Verification items for the finished model (mm, model axes). A direction names the side the tool comes from. Coordinates: 2 decimals unless noted, no trailing zeros. Loops run counter-clockwise (first coordinate to the right, second up) from the corner with the lowest first, then second, coordinate; pieces in that order, holes last. Notation, with made-up numbers: (28, 13.5) -> (43, 13.5) arc R27 cw to (43, 41.5) -> close; hole circle Ø6 at (-36, 62). An arc over 180 degrees is marked (long way). Answer as a JSON object with one key per item and string values. Group by question number.
Q1. Cross-section at D-D on z = 85.5. Record the boundary of the cut face in (x, y), and give its area (3 significant figures).
Q2. Cross-section at C-C on x = 63. Record the boundary of the cut face in (y, z).
Q3. Scan lines: L1, parallel to Y at x = 109.5, z = 40; L2, parallel to Z at x = 83, y = 8.4; L3, parallel to Z at x = 20, y = 6. Record each from-to range of solid material in increasing order.
Q4. Set-up check for faces 1 (the flat face through (72.5, 7, 76)), 2 (the flat face through (5, 47, 95)), 3 (the cylindrical face through (108, 46, 40)), 4 (the flat face through (106, 53, 8)): record each of +Z, -Z, +X, -X, +Y, -Y from which the full face is reachable in a straight line by a thin tool's end or side.
Q5. Cross-section at B-B on x = 83. Record the boundary of the cut face in (y, z).
Q6. Gauge pin test, flat ends, axial feed: pin 1 Ø1.2 at (x, y) = (4, 54) entering from -Z; pin 2 Ø1.2 at (x, y) = (107.5, 54.5) entering from +Z; pin 3 Ø8 at (x, z) = (50.5, 27.5) entering from +Y. Record the tip position at first contact, or that the pin passes through.
Q7. Cross-section at A-A on y = 38. Record the boundary of the cut face in (x, z), and give its area (3 significant figures).
Q8. Release check for a two-part mould opening along Y. For faces 5 (the cylindrical face through (108, 32, 40)), 6 (the flat face through (80, 6, 25)), 7 (the flat face through (68, 5, 13.5)), 8 (the flat face through (5, 80, 49)) record: released by +Y, released by -Y, zero draft, split by the parting line, or undercut.
```python
from build123d import *

# Parameters (mm, degrees)
BOX003_W                = 37
BOX003_H                = 7
BOX003_DEPTH            = 7
CYLINDER001_R           = 2
CYLINDER001_DEPTH       = 20
CYLINDER001_ROLL_ANGLE  = 90
ARRAY001_X_COUNT        = 2
ARRAY001_X_PITCH        = 28
ARRAY001_Z_COUNT        = 2
ARRAY001_Z_PITCH        = 50
BOX004_W                = 13
BOX004_H                = 12
BOX004_DEPTH            = 3.5
ARRAY003_X_COUNT        = 2
ARRAY003_X_PITCH        = 102
ARRAY003_Z_COUNT        = 2
ARRAY003_Z_PITCH        = 90.5
BOX002_W                = 37
BOX002_H                = 7
BOX002_DEPTH            = 7
BOX005_W                = 4
BOX005_H                = 6
BOX005_DEPTH            = 11
CYLINDER004_R           = 2
CYLINDER004_DEPTH       = 11
CYLINDER003_R           = 2
CYLINDER003_DEPTH       = 11
ARRAY004_X_COUNT        = 2
ARRAY004_X_PITCH        = 103
ARRAY004_Z_COUNT        = 2
ARRAY004_Z_PITCH        = 91
CYLINDER007_R           = 12
CYLINDER007_DEPTH       = 12
CYLINDER007_PITCH_ANGLE = 90
CYLINDER006_R           = 2.25
CYLINDER006_DEPTH       = 12
CYLINDER006_PITCH_ANGLE = 90
ARRAY006_Y_COUNT        = 2
ARRAY006_Y_PITCH        = 31
ARRAY006_Z_COUNT        = 2
ARRAY006_Z_PITCH        = 31
CYLINDER005_R           = 12
CYLINDER005_DEPTH       = 12
CYLINDER005_PITCH_ANGLE = 90
ARRAY005_Y_COUNT        = 2
ARRAY005_Y_PITCH        = 31
ARRAY005_Z_COUNT        = 2
ARRAY005_Z_PITCH        = 31
CYLINDER002_R           = 2
CYLINDER002_DEPTH       = 20
CYLINDER002_PITCH_ANGLE = 90
ARRAY002_Y_COUNT        = 4
ARRAY002_Y_PITCH        = 14
ARRAY002_Z_COUNT        = 4
ARRAY002_Z_PITCH        = 20
CYLINDER_R              = 2.5
CYLINDER_DEPTH          = 20
CYLINDER_ROLL_ANGLE     = 90
ARRAY_X_COUNT           = 2
ARRAY_X_PITCH           = 73
ARRAY_Z_COUNT           = 2
ARRAY_Z_PITCH           = 80
BOX001_W                = 8
BOX001_H                = 20
BOX001_DEPTH            = 24
BOX_W                   = 8
BOX_H                   = 20
BOX_DEPTH               = 24
EXTRUDE001_DEPTH        = 100
FILLET_R                = 1.5


with BuildPart() as h_bearing_up_h:
    # Box003 → Box003 (new body)
    with BuildSketch(Plane(origin=(50, -1, 72), x_dir=(1, 0, 0), z_dir=(0, 0, 1))):
        with Locations((18.5, 3.5)):
            Rectangle(BOX003_W, BOX003_H)
    extrude(amount=BOX003_DEPTH)


with BuildPart() as h_bearing_bolt:
    # Cylinder001 → Cylinder001 (new body)
    with BuildSketch(Plane.XY):
        Circle(CYLINDER001_R)
    extrude(amount=CYLINDER001_DEPTH)


with BuildPart() as h_bearing_bolt_1:
    # Cylinder001 roll: moved
    add(h_bearing_bolt.part.rotate(Axis((0, 0, 0), (1, 0, 0)), CYLINDER001_ROLL_ANGLE))


with BuildPart() as h_bearing_bolt_2:
    # Cylinder001 placement: moved
    add(h_bearing_bolt_1.part.moved(Location((55, 15, 25.5))))

    # Array001 X: h_bearing_bolt ×2


with BuildPart() as h_bearing_bolt_3:
    add(h_bearing_bolt_2.part)
    with Locations(*[(i * ARRAY001_X_PITCH, 0, 0) for i in range(1, ARRAY001_X_COUNT)]):
        add(h_bearing_bolt_2.part)

    # Array001 Z: h_bearing_bolt ×2


with BuildPart() as h_bearing_bolt_4:
    add(h_bearing_bolt_3.part)
    with Locations(*[(0, 0, i * ARRAY001_Z_PITCH) for i in range(1, ARRAY001_Z_COUNT)]):
        add(h_bearing_bolt_3.part)


with BuildPart() as h_nut_union001:
    # Box004 → Box004 (new body)
    with BuildSketch(Plane(origin=(-1, 47, 3), x_dir=(1, 0, 0), z_dir=(0, 0, 1))):
        with Locations((6.5, 6)):
            Rectangle(BOX004_W, BOX004_H)
    extrude(amount=BOX004_DEPTH)

    # Array003 X: h_nut_union001 ×2


with BuildPart() as h_nut_union001_1:
    add(h_nut_union001.part)
    with Locations(*[(i * ARRAY003_X_PITCH, 0, 0) for i in range(1, ARRAY003_X_COUNT)]):
        add(h_nut_union001.part)

    # Array003 Z: h_nut_union001 ×2


with BuildPart() as h_nut_union001_2:
    add(h_nut_union001_1.part)
    with Locations(*[(0, 0, i * ARRAY003_Z_PITCH) for i in range(1, ARRAY003_Z_COUNT)]):
        add(h_nut_union001_1.part)


with BuildPart() as h_bearing_dn_h:
    # Box002 → Box002 (new body)
    with BuildSketch(Plane(origin=(50, -1, 22), x_dir=(1, 0, 0), z_dir=(0, 0, 1))):
        with Locations((18.5, 3.5)):
            Rectangle(BOX002_W, BOX002_H)
    extrude(amount=BOX002_DEPTH)


with BuildPart() as h_bolt_union002:
    # Box005 → Box005 (new body)
    with BuildSketch(Plane(origin=(3, 50, -1), x_dir=(1, 0, 0), z_dir=(0, 0, 1))):
        with Locations((2, 3)):
            Rectangle(BOX005_W, BOX005_H)
    extrude(amount=BOX005_DEPTH)


with BuildPart() as h_bolt_union001:
    # Cylinder004 → Cylinder004 (new body)
    with BuildSketch(Plane(origin=(5, 56, -1), x_dir=(1, 0, 0), z_dir=(0, 0, 1))):
        Circle(CYLINDER004_R)
    extrude(amount=CYLINDER004_DEPTH)


with BuildPart() as h_bolt_union004:
    # Cylinder003 → Cylinder003 (new body)
    with BuildSketch(Plane(origin=(5, 50, -1), x_dir=(1, 0, 0), z_dir=(0, 0, 1))):
        Circle(CYLINDER003_R)
    extrude(amount=CYLINDER003_DEPTH)

    # Fusion: union h_bolt_union002, h_bolt_union001
    add(h_bolt_union002.part)
    add(h_bolt_union001.part)

    # Array004 X: h_bolt_union004 ×2


with BuildPart() as h_bolt_union004_1:
    add(h_bolt_union004.part)
    with Locations(*[(i * ARRAY004_X_PITCH, 0, 0) for i in range(1, ARRAY004_X_COUNT)]):
        add(h_bolt_union004.part)

    # Array004 Z: h_bolt_union004 ×2


with BuildPart() as h_bolt_union004_2:
    add(h_bolt_union004_1.part)
    with Locations(*[(0, 0, i * ARRAY004_Z_PITCH) for i in range(1, ARRAY004_Z_COUNT)]):
        add(h_bolt_union004_1.part)


with BuildPart() as h_motor_axis001:
    # Cylinder007 → Cylinder007 (new body)
    with BuildSketch(Plane.XY):
        Circle(CYLINDER007_R)
    extrude(amount=CYLINDER007_DEPTH)


with BuildPart() as h_motor_axis001_1:
    # Cylinder007 pitch: moved
    add(h_motor_axis001.part.rotate(Axis((0, 0, 0), (0, 1, 0)), CYLINDER007_PITCH_ANGLE))


with BuildPart() as h_motor_axis001_2:
    # Cylinder007 placement: moved
    add(h_motor_axis001_1.part.moved(Location((-1, 60, 25))))


with BuildPart() as h_bolt_motor:
    # Cylinder006 → Cylinder006 (new body)
    with BuildSketch(Plane.XY):
        Circle(CYLINDER006_R)
    extrude(amount=CYLINDER006_DEPTH)


with BuildPart() as h_bolt_motor_1:
    # Cylinder006 pitch: moved
    add(h_bolt_motor.part.rotate(Axis((0, 0, 0), (0, 1, 0)), CYLINDER006_PITCH_ANGLE))


with BuildPart() as h_bolt_motor_2:
    # Cylinder006 placement: moved
    add(h_bolt_motor_1.part.moved(Location((-1, 44.5, 9.5))))


with BuildPart() as h_holes_motor_dn:
    # Array006 base: copy of h_bolt_motor
    add(h_bolt_motor_2.part)

    # Array006 Y: h_holes_motor_dn ×2


with BuildPart() as h_holes_motor_dn_1:
    add(h_holes_motor_dn.part)
    with Locations(*[(0, i * ARRAY006_Y_PITCH, 0) for i in range(1, ARRAY006_Y_COUNT)]):
        add(h_holes_motor_dn.part)

    # Array006 Z: h_holes_motor_dn ×2


with BuildPart() as h_holes_motor_dn_2:
    add(h_holes_motor_dn_1.part)
    with Locations(*[(0, 0, i * ARRAY006_Z_PITCH) for i in range(1, ARRAY006_Z_COUNT)]):
        add(h_holes_motor_dn_1.part)

    # Fusion002: union h_motor_axis001
    add(h_motor_axis001_2.part)


with BuildPart() as h_motor_axis:
    # Cylinder005 → Cylinder005 (new body)
    with BuildSketch(Plane.XY):
        Circle(CYLINDER005_R)
    extrude(amount=CYLINDER005_DEPTH)


with BuildPart() as h_motor_axis_1:
    # Cylinder005 pitch: moved
    add(h_motor_axis.part.rotate(Axis((0, 0, 0), (0, 1, 0)), CYLINDER005_PITCH_ANGLE))


with BuildPart() as h_motor_axis_2:
    # Cylinder005 placement: moved
    add(h_motor_axis_1.part.moved(Location((-1, 60, 25))))


with BuildPart() as h_holes_motor_up:
    # Array005 base: copy of h_bolt_motor
    add(h_bolt_motor_2.part)

    # Array005 Y: h_holes_motor_up ×2


with BuildPart() as h_holes_motor_up_1:
    add(h_holes_motor_up.part)
    with Locations(*[(0, i * ARRAY005_Y_PITCH, 0) for i in range(1, ARRAY005_Y_COUNT)]):
        add(h_holes_motor_up.part)

    # Array005 Z: h_holes_motor_up ×2


with BuildPart() as h_holes_motor_up_2:
    add(h_holes_motor_up_1.part)
    with Locations(*[(0, 0, i * ARRAY005_Z_PITCH) for i in range(1, ARRAY005_Z_COUNT)]):
        add(h_holes_motor_up_1.part)

    # Fusion001: union h_motor_axis
    add(h_motor_axis_2.part)


with BuildPart() as h_holes_motor_up_3:
    # Fusion001 placement: moved
    add(h_holes_motor_up_2.part.moved(Location((0, 0, 50))))


with BuildPart() as h_front_holes:
    # Cylinder002 → Cylinder002 (new body)
    with BuildSketch(Plane.XY):
        Circle(CYLINDER002_R)
    extrude(amount=CYLINDER002_DEPTH)


with BuildPart() as h_front_holes_1:
    # Cylinder002 pitch: moved
    add(h_front_holes.part.rotate(Axis((0, 0, 0), (0, 1, 0)), CYLINDER002_PITCH_ANGLE))


with BuildPart() as h_front_holes_2:
    # Cylinder002 placement: moved
    add(h_front_holes_1.part.moved(Location((100, 20, 20))))

    # Array002 Y: h_front_holes ×4


with BuildPart() as h_front_holes_3:
    add(h_front_holes_2.part)
    with Locations(*[(0, i * ARRAY002_Y_PITCH, 0) for i in range(1, ARRAY002_Y_COUNT)]):
        add(h_front_holes_2.part)

    # Array002 Z: h_front_holes ×4


with BuildPart() as h_front_holes_4:
    add(h_front_holes_3.part)
    with Locations(*[(0, 0, i * ARRAY002_Z_PITCH) for i in range(1, ARRAY002_Z_COUNT)]):
        add(h_front_holes_3.part)


with BuildPart() as h_holes_extra_up:
    # Cylinder → Cylinder (new body)
    with BuildSketch(Plane.XY):
        Circle(CYLINDER_R)
    extrude(amount=CYLINDER_DEPTH)


with BuildPart() as h_holes_extra_up_1:
    # Cylinder roll: moved
    add(h_holes_extra_up.part.rotate(Axis((0, 0, 0), (1, 0, 0)), CYLINDER_ROLL_ANGLE))


with BuildPart() as h_holes_extra_up_2:
    # Cylinder placement: moved
    add(h_holes_extra_up_1.part.moved(Location((20, 15, 10))))

    # Array X: h_holes_extra_up ×2


with BuildPart() as h_holes_extra_up_3:
    add(h_holes_extra_up_2.part)
    with Locations(*[(i * ARRAY_X_PITCH, 0, 0) for i in range(1, ARRAY_X_COUNT)]):
        add(h_holes_extra_up_2.part)

    # Array Z: h_holes_extra_up ×2


with BuildPart() as h_holes_extra_up_4:
    add(h_holes_extra_up_3.part)
    with Locations(*[(0, 0, i * ARRAY_Z_PITCH) for i in range(1, ARRAY_Z_COUNT)]):
        add(h_holes_extra_up_3.part)


with BuildPart() as h_bearing_dn_v:
    # Box001 → Box001 (new body)
    with BuildSketch(Plane(origin=(64.5, -5, 13.5), x_dir=(1, 0, 0), z_dir=(0, 0, 1))):
        with Locations((4, 10)):
            Rectangle(BOX001_W, BOX001_H)
    extrude(amount=BOX001_DEPTH)


with BuildPart() as holes:
    # Box → Box (new body)
    with BuildSketch(Plane(origin=(64.5, -5, 64), x_dir=(1, 0, 0), z_dir=(0, 0, 1))):
        with Locations((4, 10)):
            Rectangle(BOX_W, BOX_H)
    extrude(amount=BOX_DEPTH)

    # Fusion003: union h_bearing_up_h, h_bearing_bolt, h_nut_union001, h_bearing_dn_h, h_bolt_union004, h_holes_motor_dn, h_holes_motor_up, h_front_holes, h_holes_extra_up, h_bearing_dn_v
    add(h_bearing_up_h.part)
    add(h_bearing_bolt_4.part)
    add(h_nut_union001_2.part)
    add(h_bearing_dn_h.part)
    add(h_bolt_union004_2.part)
    add(h_holes_motor_dn_2.part)
    add(h_holes_motor_up_3.part)
    add(h_front_holes_4.part)
    add(h_holes_extra_up_4.part)
    add(h_bearing_dn_v.part)


with BuildPart() as fillet_body:
    # Sketch → Extrude001 (new body)
    with BuildSketch(Plane.XY):
        Polygon((-56.5, 80), (-46.5, 80), (-46.5, 10), (46.5, 10), (46.5, 80), (56.5, 80), (56.5, 0), (-56.5, 0), align=None)
    extrude(amount=EXTRUDE001_DEPTH)


with BuildPart() as fillet_body_1:
    # Extrude001 placement: moved
    add(fillet_body.part.moved(Location((56.5, 0, 0))))

    # Cut: cut holes
    add(holes.part, mode=Mode.SUBTRACT)

    # Fillet
    fillet_edges = [fillet_body_1.edges().sort_by_distance(p)[0] for p in [
        (0, 80, 50),
        (10, 80, 50),
        (5, 80, 0),
        (5, 80, 100),
        (0, 0, 50),
        (0, 40, 0),
        (0, 40, 100),
        (10, 45, 0),
        (10, 45, 100),
        (10, 10, 50),
        (56.5, 0, 0),
        (56.5, 10, 0),
        (113, 40, 0),
        (103, 45, 0),
        (108, 80, 0),
        (56.5, 0, 100),
        (56.5, 10, 100),
        (113, 40, 100),
        (103, 45, 100),
        (108, 80, 100),
        (113, 0, 50),
        (103, 10, 50),
        (113, 80, 50),
        (103, 80, 50),
    ]]
    fillet(fillet_edges, radius=FILLET_R)


solid = fillet_body_1.part
```
Computed values:
{
 "1": {"outline": "(0, 1.5) arc R1.5 ccw to (1.5, 0) -> (64.5, 0) -> (64.5, 10) -> (11.5, 10) arc R1.5 cw to (10, 11.5) -> (10, 54.19) -> (0, 54.19) -> close; (0, 65.81) -> (10, 65.81) -> (10, 78.5) arc R1.5 ccw to (8.5, 80) -> (1.5, 80) arc R1.5 ccw to (0, 78.5) -> close; (72.5, 0) -> (111.5, 0) arc R1.5 ccw to (113, 1.5) -> (113, 78.5) arc R1.5 ccw to (111.5, 80) -> (104.5, 80) arc R1.5 ccw to (103, 78.5) -> (103, 11.5) arc R1.5 cw to (101.5, 10) -> (72.5, 10) -> close", "area": "2,330 mm²"},
 "2": {"outline": "(0, 1.5) arc R1.5 ccw to (1.5, 0) -> (8.5, 0) arc R1.5 ccw to (10, 1.5) -> (10, 98.5) arc R1.5 ccw to (8.5, 100) -> (1.5, 100) arc R1.5 ccw to (0, 98.5) -> (0, 79) -> (6, 79) -> (6, 72) -> (0, 72) -> (0, 29) -> (6, 29) -> (6, 22) -> (0, 22) -> close"},
 "3": {"L1": "y = 0 to 18, 22 to 32, 36 to 46, 50 to 60, 64 to 80", "L2": "z = 0 to 23.5, 27.5 to 73.5, 77.5 to 100", "L3": "z = 0 to 7.5, 12.5 to 87.5, 92.5 to 100"},
 "4": {"face 1": "+Y, -Y", "face 2": "+X, -X", "face 3": "+X", "face 4": "-Z"},
 "5": {"outline": "(0, 1.5) arc R1.5 ccw to (1.5, 0) -> (8.5, 0) arc R1.5 ccw to (10, 1.5) -> (10, 23.5) -> (6, 23.5) -> (6, 22) -> (0, 22) -> close; (0, 29) -> (6, 29) -> (6, 27.5) -> (10, 27.5) -> (10, 73.5) -> (6, 73.5) -> (6, 72) -> (0, 72) -> close; (0, 79) -> (6, 79) -> (6, 77.5) -> (10, 77.5) -> (10, 98.5) arc R1.5 ccw to (8.5, 100) -> (1.5, 100) arc R1.5 ccw to (0, 98.5) -> close"},
 "6": {"pin 1": "stops at z = 10", "pin 2": "stops at z = 90", "pin 3": "stops at y = 10"},
 "7": {"outline": "(0, 1.5) arc R1.5 ccw to (1.5, 0) -> (8.5, 0) arc R1.5 ccw to (10, 1.5) -> (10, 98.5) arc R1.5 ccw to (8.5, 100) -> (1.5, 100) arc R1.5 ccw to (0, 98.5) -> close; (103, 1.5) arc R1.5 ccw to (104.5, 0) -> (111.5, 0) arc R1.5 ccw to (113, 1.5) -> (113, 98.5) arc R1.5 ccw to (111.5, 100) -> (104.5, 100) arc R1.5 ccw to (103, 98.5) -> close", "area": "2,000 mm²"},
 "8": {"face 5": "undercut", "face 6": "released by -Y", "face 7": "zero draft", "face 8": "released by +Y"}
}
